```python
from build123d import *

# Parameters (mm, degrees)
BOSS_EXTRUDE2_START     = -0.2
BOSS_EXTRUDE2_DEPTH     = 1.63
SKETCH5_W               = 0.7
SKETCH5_H               = 1
BOSS_EXTRUDE4_DEPTH     = 0.7
SKETCH6_W               = 0.4
SKETCH6_H               = 1
BOSS_EXTRUDE5_DEPTH     = 0.7
CUT_EXTRUDE1_DEPTH      = 0.7
CUT_EXTRUDE1_DEPTH_BACK = 3.33
SKETCH7_R               = 0.25
CUT_EXTRUDE2_DEPTH      = 8.827352199


with BuildPart() as part:
    # Sketch2 → Boss-Extrude2 (new body)
    with BuildSketch(Plane.XY.offset(BOSS_EXTRUDE2_START)):
        Polygon((-0.5, 2.16), (-0.5, -4.7), (0.1, -4.7), (0.1, -5.000793217), (-0.694374061, -5.667352199), (-1.2, -5.667352199), (-1.2, 2.16), align=None)
    extrude(amount=-BOSS_EXTRUDE2_DEPTH)

    # Sketch5 → Boss-Extrude4 (add)
    with BuildSketch(Plane.XY.offset(-0.2)):
        with Locations((-0.85, 1.66)):
            Rectangle(SKETCH5_W, SKETCH5_H)
    boss_extrude4 = extrude(amount=BOSS_EXTRUDE4_DEPTH)

    # Sketch6 → Boss-Extrude5 (add)
    with BuildSketch(Plane(origin=(-0.5, 0, 0), x_dir=(0, 0, -1), z_dir=(1, 0, 0))):
        with Locations((-0.3, 1.66)):
            Rectangle(SKETCH6_W, SKETCH6_H)
    boss_extrude5 = extrude(amount=BOSS_EXTRUDE5_DEPTH)

    # Mirror1: Boss-Extrude4, Boss-Extrude5 across plane
    add(boss_extrude4.mirror(Plane.XY.offset(-1.015)))
    add(boss_extrude5.mirror(Plane.XY.offset(-1.015)))

    # Sketch3 → Cut-Extrude1 (cut, two sides)
    with BuildSketch(Plane.XY.offset(-0.2)) as cut_extrude1_sk:
        Polygon((-0.85, 2.16), (-1.2, -2.2536761), (-1.2, 2.16), align=None)
    extrude(amount=CUT_EXTRUDE1_DEPTH, mode=Mode.SUBTRACT)
    extrude(cut_extrude1_sk.sketch, amount=-CUT_EXTRUDE1_DEPTH_BACK, mode=Mode.SUBTRACT)

    # Sketch7 → Cut-Extrude2 (cut, through all)
    with BuildSketch(Plane(origin=(0, 2.16, 0), x_dir=(1, 0, 0), z_dir=(0, 1, 0))):
        with Locations((-0.85, 1.015)):
            Circle(SKETCH7_R)
    extrude(amount=-CUT_EXTRUDE2_DEPTH, mode=Mode.SUBTRACT)


solid = part.part
```
Here's how the part is built. I have some questions about the finished solid (model axes, mm). A direction names the side the tool comes from. Round coordinates to 2 decimals unless told otherwise and drop trailing zeros. Order: outer loops, then holes, each group sorted by start corner. A loop starts at its lowest first (then second) coordinate and runs counter-clockwise, first axis right, second up. Notation, with made-up numbers: M 45,-33 L 56,-33 A22 cw 56,-21 Z; hole C 26.5,28.5 d4. An arc over 180 degrees is marked long. Answer in a Markdown table with one row per item.
Item 1: Imagine slicing it at A-A, the plane x = -0.3. Write out the boundary of the cut face in (y, z), and give its area (3 significant figures).
A:
| item | result |
|---|---|
| outline | M -5.34,-1.83 L -4.7,-1.83 L -4.7,-0.2 L -5.34,-0.2 Z; M 1.16,-2.53 L 2.16,-2.53 L 2.16,-2.13 L 1.16,-2.13 Z; M 1.16,0.1 L 2.16,0.1 L 2.16,0.5 L 1.16,0.5 Z |
| area | 1.84 mm2 |
Item 2: If I drill on L1, parallel to Z at x = -0.85, y = 0.75 (3 decimals); L2, parallel to X at y = -4.5, z = -0.3; L3, parallel to X at y = -1, z = -1.3, over which ranges is the centre line in solid material (lowest first)? Write a range as from..to.
A:
| item | result |
|---|---|
| L1 | z = -1.83..-1.265, -0.765..-0.2 |
| L2 | x = -1.2..-0.5 |
| L3 | x = -1.1..-0.5 |
Item 3: For faces 1 (the face through (-0.5, -1.3, -0.8)), 2 (the face through (-1, -2, -0.2)), 3 (the face through (-1, -2, -1.83)), which set-ups out of +Z, -Z, +X, -X, +Y, -Y let a thin tool reach every point of the face, with its end or its side?
A:
| item | result |
|---|---|
| face 1 | +X, +Y |
| face 2 | +Z, +X, -X, -Y |
| face 3 | -Z, +X, -X, -Y |
Item 4: Imagine slicing it at B-B, the plane z = -1.5. Write out the boundary of the cut face in (x, y), and give its area (3 significant figures).
A:
| item | result |
|---|---|
| outline | M -1.2,-5.67 L -0.69,-5.67 L 0.1,-5 L 0.1,-4.7 L -0.5,-4.7 L -0.5,2.16 L -0.85,2.16 L -1.2,-2.25 Z |
| area | 5.02 mm2 |
Item 5: Imagine slicing it at D-D, the plane y = -2.5. Write out the boundary of the cut face in (x, z) (3 decimals).
A:
| item | result |
|---|---|
| outline | M -1.2,-1.83 L -0.5,-1.83 L -0.5,-0.2 L -1.2,-0.2 Z; hole C -0.85,-1.015 d0.5 |
Item 6: I'm going to push flat-ended pins straight in: pin 1 (1.8 mm diameter, centred on y = -1.5, z = -0.5, fed in from +X); pin 2 (0.6 mm diameter, centred on x = -1, y = -3.5, fed in from -Z); pin 3 (0.8 mm diameter, centred on x = -0.5, z = 0.5, fed in from -Y). Where does each tip first touch, or does it pass through?
A:
| item | result |
|---|---|
| pin 1 | stops at x = -0.5 |
| pin 2 | stops at z = -1.83 |
| pin 3 | stops at y = 1.16 |
Item 7: Imagine slicing it at C-C, the plane z = -1.1. Write out the boundary of the cut face in (x, y).
A:
| item | result |
|---|---|
| outline | M -1.2,-5.67 L -1.09,-5.67 L -1.09,-0.8 L -1.2,-2.25 Z; M -0.61,-5.6 L 0.1,-5 L 0.1,-4.7 L -0.5,-4.7 L -0.5,2.16 L -0.61,2.16 Z |
